The model under review builds one solid part; all positions refer to its coordinate system, in mm. Coordinates: 2 decimals unless noted, no trailing zeros. Write each loop counter-clockwise with the first axis right and the second up, starting at its lowest first coordinate (ties: lowest second). Pieces come first, ordered by that corner, then holes.
1) Add section A-A, the plane y = 327.5. State the section outline as (x, z) points.
2) For line 1 (X direction, y = -439.25, z = 7); line 2 (Z direction, x = 20.5, y = -147.5); line 3 (X direction, y = -439.25, z = -7), list the stretches that pass through material, from the lowest coordinate up.
3) For P1, Ø5, axis at x = -10.5, z = -6.5, coming from the -Y side; P2, Ø4.5, axis at x = 2.5, y = -111.5, coming from the +Z side; P3, Ø4, axis at x = 19.5, z = -7, coming from the -Y side; P4, Ø12, axis at x = 8.5, z = 7, coming from the -Y side, all flat-tipped, find the tip position at first contact; note any pin that passes through.
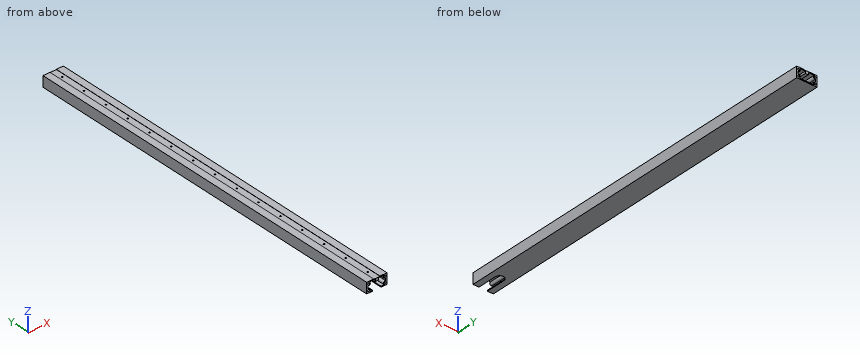
from build123d import *

# Parameters (mm, degrees)
SKETCH_1_W             = 48
SKETCH_1_H             = 25
EXTRUDE_1_DEPTH        = 445
SKETCH_2_R             = 1.9
CUT_EXTRUDE_1_DEPTH    = 891.411281375
SKETCH_3_W             = 15
SKETCH_3_H             = 0.5
CUT_EXTRUDE_2_DEPTH    = 891.411281375
PATTERN_LINEAR_1_COUNT = 15
PATTERN_LINEAR_1_PITCH = 60
CUT_EXTRUDE_3_DEPTH    = 2
M5X0_8_1_AT_2_COUNT    = 2
M5X0_8_1_AT_2_PITCH    = 14
M5X0_8_1_AT_3_COUNT    = 2
M5X0_8_1_AT_3_PITCH    = 39
M5X0_8_1_AT_4_COUNT    = 2
M5X0_8_1_AT_4_PITCH    = 41.43669871


with BuildPart() as part:
    # 草图1 → 凸台-拉伸1 (new, symmetric)
    with BuildSketch(Plane(origin=(0, 0, 0), x_dir=(1, 0, 0), z_dir=(0, 1, 0))):
        Rectangle(SKETCH_1_W, SKETCH_1_H)
    extrude(amount=EXTRUDE_1_DEPTH, both=True)

    # 草图2 → 切除-拉伸1 (cut, through all)
    with BuildSketch(Plane.XZ.offset(445)):
        with Locations(Location((-19.5, 7, 0), (0, 0, 270))):
            Circle(SKETCH_2_R)
        with Locations(Location((-19.5, -7, 0), (0, 0, 90))):
            Circle(SKETCH_2_R)
        with Locations(Location((19.5, -7, 0), (0, 0, 270))):
            Circle(SKETCH_2_R)
        with Locations(Location((19.5, 7, 0), (0, 0, 90))):
            Circle(SKETCH_2_R)
        with BuildLine():
            Line((-17.563508327, 10.5), (-3.5, 10.5))
            Line((-3.5, 10.5), (-3.5, 5.5))
            Line((-3.5, 5.5), (3.5, 5.5))
            Line((3.5, 5.5), (3.5, 10.5))
            Line((3.5, 10.5), (17.563508327, 10.5))
            ThreePointArc((17.563508327, 10.5), (15.889348408, 5.278606646), (21, 3.291900756))
            Line((21, 3.291900756), (21, -3.291900756))
            ThreePointArc((21, -3.291900756), (15.889348408, -5.278606646), (17.563508327, -10.5))
            Line((17.563508327, -10.5), (-17.563508327, -10.5))
            ThreePointArc((-17.563508327, -10.5), (-15.889348408, -5.278606646), (-21, -3.291900756))
            Line((-21, -3.291900756), (-21, 3.291900756))
            ThreePointArc((-21, 3.291900756), (-15.889348408, 5.278606646), (-17.563508327, 10.5))
        make_face()
    extrude(amount=-CUT_EXTRUDE_1_DEPTH, mode=Mode.SUBTRACT)

    # 草图3 → 切除-拉伸2 (cut, through all)
    with BuildSketch(Plane.XZ.offset(445)):
        with Locations((0, 12.25)):
            Rectangle(SKETCH_3_W, SKETCH_3_H)
    extrude(amount=-CUT_EXTRUDE_2_DEPTH, mode=Mode.SUBTRACT)

    # 草图4 → M4x0.7 螺纹孔1 (revolve, cut)
    with BuildSketch(Plane(origin=(0, 420, 12), x_dir=(0, -1, 0), z_dir=(1, 0, 0))):
        Polygon((0, 0), (0, 11.091420021), (1.65, 10.1), (1.65, 0), align=None)
    m4x0_7_1 = revolve(axis=Axis((0, 420, 18.35), (0, 0, -1)), mode=Mode.SUBTRACT)

    # 阵列(线性)1: M4x0.7 螺纹孔1 ×15
    with Locations(*[(0, -i * PATTERN_LINEAR_1_PITCH, 0) for i in range(1, PATTERN_LINEAR_1_COUNT)]):
        add(m4x0_7_1, mode=Mode.SUBTRACT)

    # 草图6 → 切除-拉伸3 (cut)
    with BuildSketch(Plane(origin=(0, 0, -12.5), x_dir=(-1, 0, 0), z_dir=(0, 0, -1))):
        with BuildLine():
            Line((10, -400), (10, -445))
            ThreePointArc((10, -445), (0, -455), (-10, -445))
            Line((-10, -445), (-10, -400))
            ThreePointArc((-10, -400), (0, -390), (10, -400))
        make_face()
    extrude(amount=-CUT_EXTRUDE_3_DEPTH, mode=Mode.SUBTRACT)

    # 草图7 → M5x0.8 螺纹孔1 (revolve, cut)
    with BuildSketch(Plane(origin=(-19.5, 445, -7), x_dir=(0, 0, 1), z_dir=(1, 0, 0))):
        Polygon((0, 0), (0, 13.6618073), (2.1, 12.4), (2.1, 0), align=None)
    m5x0_8_1 = revolve(axis=Axis((-19.5, 451.35, -7), (0, -1, 0)), mode=Mode.SUBTRACT)

    # M5x0.8 螺纹孔1 at 2: M5x0.8 螺纹孔1 ×2
    with Locations(*[(0, 0, i * M5X0_8_1_AT_2_PITCH) for i in range(1, M5X0_8_1_AT_2_COUNT)]):
        add(m5x0_8_1, mode=Mode.SUBTRACT)

    # M5x0.8 螺纹孔1 at 3: M5x0.8 螺纹孔1 ×2
    with Locations(*[(i * M5X0_8_1_AT_3_PITCH, 0, 0) for i in range(1, M5X0_8_1_AT_3_COUNT)]):
        add(m5x0_8_1, mode=Mode.SUBTRACT)

    # M5x0.8 螺纹孔1 at 4: M5x0.8 螺纹孔1 ×2
    with Locations(*[Vector(0.9411946707617075, 0, 0.33786475360676677) * (i * M5X0_8_1_AT_4_PITCH) for i in range(1, M5X0_8_1_AT_4_COUNT)]):
        add(m5x0_8_1, mode=Mode.SUBTRACT)

    # 镜向1: M5x0.8 螺纹孔1 across plane
    add(m5x0_8_1.mirror(Plane.ZX), mode=Mode.SUBTRACT)

    # 镜向1 copy 1 sketch → 镜向1 copy 1 (revolve, cut)
    with BuildSketch(Plane(origin=(-19.5, -445, 7), x_dir=(0, 0, 1), z_dir=(1, 0, 0))):
        Polygon((0, 0), (0, -13.6618073), (2.1, -12.4), (2.1, 0), align=None)
    revolve(axis=Axis((-19.5, -451.35, 7), (0, -1, 0)), mode=Mode.SUBTRACT)

    # 镜向1 copy 2 sketch → 镜向1 copy 2 (revolve, cut)
    with BuildSketch(Plane(origin=(19.5, -445, -7), x_dir=(0, 0, 1), z_dir=(1, 0, 0))):
        Polygon((0, 0), (0, -13.6618073), (2.1, -12.4), (2.1, 0), align=None)
    revolve(axis=Axis((19.5, -451.35, -7), (0, -1, 0)), mode=Mode.SUBTRACT)

    # 镜向1 copy 3 sketch → 镜向1 copy 3 (revolve, cut)
    with BuildSketch(Plane(origin=(19.5, -445, 7), x_dir=(0, 0, 1), z_dir=(1, 0, 0))):
        Polygon((0, 0), (0, -13.6618073), (2.1, -12.4), (2.1, 0), align=None)
    revolve(axis=Axis((19.5, -451.35, 7), (0, -1, 0)), mode=Mode.SUBTRACT)


solid = part.part
Geometry results:
1. outline: (-24, -12.5) - (24, -12.5) - (24, 12.5) - (7.5, 12.5) - (7.5, 12) - (-7.5, 12) - (-7.5, 12.5) - (-24, 12.5) - close; hole circle Ø3.8 at (-19.5, -7); hole circle Ø3.8 at (-19.5, 7); hole (-21, -3.29) arc R4 cw to (-17.56, -10.5) - (17.56, -10.5) arc R4 cw to (21, -3.29) - (21, 3.29) arc R4 cw to (17.56, 10.5) - (3.5, 10.5) - (3.5, 5.5) - (-3.5, 5.5) - (-3.5, 10.5) - (-17.56, 10.5) arc R4 cw to (-21, 3.29) - close; hole circle Ø3.8 at (19.5, -7); hole circle Ø3.8 at (19.5, 7)
2. line 1: x = -24 to -21.6, -17.4 to -15.5, -3.5 to 3.5, 15.5 to 17.4, 21.6 to 24
2. line 2: z = -12.5 to -8.62, -5.38 to -3.13, 3.13 to 5.38, 8.62 to 12.5
2. line 3: x = -24 to -21.6, -17.4 to -15.5, 15.5 to 17.4, 21.6 to 24
3. P1: passes through
3. P2: stops at z = 12
3. P3: stops at y = -432.54
3. P4: stops at y = -445
